```python
from build123d import *

# Parameters (mm, degrees)
SKETCH1_W                                           = 50
SKETCH1_H                                           = 50
BOSS_EXTRUDE1_DEPTH                                 = 34
CBORE_FOR_M4_HEX_SOCKET_HEAD_CAP_SCREW1_D           = 4.5
CBORE_FOR_M4_HEX_SOCKET_HEAD_CAP_SCREW1_CBORE_D     = 8
CBORE_FOR_M4_HEX_SOCKET_HEAD_CAP_SCREW1_CBORE_DEPTH = 4.4
SKETCH6_R                                           = 10
CUT_EXTRUDE1_DEPTH                                  = 35


with BuildPart() as part:
    # Sketch1 → Boss-Extrude1 (new body)
    with BuildSketch(Plane.XY):
        Rectangle(SKETCH1_W, SKETCH1_H)
    extrude(amount=BOSS_EXTRUDE1_DEPTH)

    # CBORE for M4 Hex Socket Head Cap Screw1 (through all)
    with Locations(Plane(origin=(0, 25, 0), x_dir=(1, 0, 0), z_dir=(0, 1, 0))):
        with Locations((-20, -5), (20, -5), (20, -29), (-20, -29)):
            CounterBoreHole(CBORE_FOR_M4_HEX_SOCKET_HEAD_CAP_SCREW1_D / 2, CBORE_FOR_M4_HEX_SOCKET_HEAD_CAP_SCREW1_CBORE_D / 2, CBORE_FOR_M4_HEX_SOCKET_HEAD_CAP_SCREW1_CBORE_DEPTH)

    # Sketch6 → Cut-Extrude1 (cut, through all)
    with BuildSketch(Plane.XY.offset(34)):
        Circle(SKETCH6_R)
    extrude(amount=-CUT_EXTRUDE1_DEPTH, mode=Mode.SUBTRACT)


solid = part.part
```
Part model, mm, in its own coordinate system. A direction names the side the tool comes from. Round coordinates to 2 decimals unless told otherwise and drop trailing zeros. Write each loop counter-clockwise with the first axis right and the second up, starting at its lowest first coordinate (ties: lowest second). Pieces come first, ordered by that corner, then holes. Notation, with made-up numbers: (20.5, 18) -> (54.5, 18) arc R14 cw to (54.5, 24) -> close; hole circle Ø7 at (10.25, -2.5). An arc over 180 degrees is marked (long way). Return JSON: item names as keys, results as strings. Group by question number.
Q1. Saw through at C-C on x = -20. Write the cut outline in (y, z), plus the area to 3 significant figures.
Q2. Mould opens along X. For faces 1 (the flat face through (-25, 0, 17)), 2 (the flat face through (0, 11, 34)), 3 (the cylindrical face through (16.8, 22.8, 7.4)) say: pulls with the +X half, pulls with the -X half, needs draft (parallel to the pull), parting line crosses it, or undercut.
Q3. Probe L1, parallel to Z at x = -20, y = 2; L2, parallel to X at y = 21.6, z = 29; L3, parallel to Z at x = 20, y = 21.7. List the from-to ranges inside material, lowest first. Write a range as [from, to].
Q4. Saw through at B-B on z = 5. Write the cut outline in (x, y), plus the area to 3 significant figures.
Q5. Pin check, flat tip, straight feed: pin 1 (4 mm diameter, centred on x = -20, z = 4, fed in from +Y). Stop position of the tip, or through.
Q6. Which spindle directions (+Z, -Z, +X, -X, +Y, -Y) get a long thin tool onto all of the face, cutting with end or side? Do faces 4 (the cylindrical face through (-20.521, 22.831, 25.034)), 5 (the flat face through (0, 11, 0)). Say none if no direction does.
Q7. Saw through at A-A on y = 8. Write the cut outline in (x, z), plus the area to 3 significant figures.
Q8. Saw through at D-D on x = 0. Write the cut outline in (y, z).
Answer:
{
 "1": {"outline": "(-25, 0) -> (25, 0) -> (25, 1) -> (20.6, 1) -> (20.6, 2.75) -> (-25, 2.75) -> close; (-25, 7.25) -> (20.6, 7.25) -> (20.6, 9) -> (25, 9) -> (25, 25) -> (20.6, 25) -> (20.6, 26.75) -> (-25, 26.75) -> close; (-25, 31.25) -> (20.6, 31.25) -> (20.6, 33) -> (25, 33) -> (25, 34) -> (-25, 34) -> close", "area": "1,220 mm2"},
 "2": {"face 1": "pulls with the -X half", "face 2": "needs draft", "face 3": "undercut"},
 "3": {"L1": "[0, 2.75], [7.25, 26.75], [31.25, 34]", "L2": "[-25, -24], [-16, 16], [24, 25]", "L3": "[0, 1], [9, 25], [33, 34]"},
 "4": {"outline": "(-25, -25) -> (-22.25, -25) -> (-22.25, 20.6) -> (-24, 20.6) -> (-24, 25) -> (-25, 25) -> close; (-17.75, -25) -> (17.75, -25) -> (17.75, 20.6) -> (16, 20.6) -> (16, 25) -> (-16, 25) -> (-16, 20.6) -> (-17.75, 20.6) -> close; (22.25, -25) -> (25, -25) -> (25, 25) -> (24, 25) -> (24, 20.6) -> (22.25, 20.6) -> close; hole circle Ø20 at (0, 0)", "area": "1,710 mm2"},
 "5": {"pin 1": "y = 20.6"},
 "6": {"face 4": "+Y", "face 5": "-Z, +X, -X, +Y, -Y"},
 "7": {"outline": "(-25, 0) -> (-6, 0) -> (-6, 34) -> (-25, 34) -> close; (6, 0) -> (25, 0) -> (25, 34) -> (6, 34) -> close; hole circle Ø4.5 at (-20, 5); hole circle Ø4.5 at (-20, 29); hole circle Ø4.5 at (20, 5); hole circle Ø4.5 at (20, 29)", "area": "1,230 mm2"},
 "8": {"outline": "(-25, 0) -> (-10, 0) -> (-10, 34) -> (-25, 34) -> close; (10, 0) -> (25, 0) -> (25, 34) -> (10, 34) -> close"}
}
